Verification items for the finished model (mm, model axes). Round coordinates to 2 decimals unless told otherwise and drop trailing zeros. Order: outer loops, then holes, each group sorted by start corner. A loop starts at its lowest first (then second) coordinate and runs counter-clockwise, first axis right, second up. Notation, with made-up numbers: M 86.25,-12.5 L 113.25,-12.5 A22 ccw 113.25,3.5 Z; hole C 52.5,14 d9. An arc over 180 degrees is marked long. One line per item, written item: value. Start each with the question number.
from build123d import *

# Parameters (mm, degrees)
SKETCH_W             = 129
SKETCH_H             = 90
PAD_DEPTH            = 2
SKETCH001_R          = 2.5
POCKET_DEPTH         = 2.001
SKETCH002_R          = 4.375
POCKET001_DEPTH      = 0.02
SKETCH003_R          = 3.25
PAD001_DEPTH         = 8.2
PAD001_DEPTH_BACK    = -2
POCKET002_DEPTH      = 10
POCKET002_DEPTH_BACK = -5
SKETCH005_W          = 3.16625
SKETCH005_H          = 2
POCKET003_DEPTH      = 45.001
POCKET004_DEPTH      = 53.251


with BuildPart() as part:
    # Sketch → Pad (new body)
    with BuildSketch(Plane.XZ):
        Rectangle(SKETCH_W, SKETCH_H)
    extrude(amount=PAD_DEPTH)

    # Sketch001 → Pocket (cut, through all)
    with BuildSketch(Plane.XZ):
        with Locations((55, 40)):
            Circle(SKETCH001_R)
        with Locations((-55, 40)):
            Circle(SKETCH001_R)
        with Locations((55, -40)):
            Circle(SKETCH001_R)
        with Locations((-55, -40)):
            Circle(SKETCH001_R)
    extrude(amount=POCKET_DEPTH, mode=Mode.SUBTRACT)

    # Sketch002 → Pocket001 (cut)
    with BuildSketch(Plane.XZ):
        with Locations((55, 40)):
            Circle(SKETCH002_R)
        with Locations((-55, 40)):
            Circle(SKETCH002_R)
        with Locations((55, -40)):
            Circle(SKETCH002_R)
        with Locations((-55, -40)):
            Circle(SKETCH002_R)
    extrude(amount=POCKET001_DEPTH, mode=Mode.SUBTRACT)

    # Sketch003 → Pad001 (join, two sides)
    with BuildSketch(Plane.XZ) as pad001_sk:
        with Locations((-15, 40)):
            Circle(SKETCH003_R)
        with BuildLine():
            ThreePointArc((24.25, 50), (21, 53.25), (17.75, 50))
            Line((17.75, 50), (17.75, 40))
            ThreePointArc((17.75, 40), (21, 36.75), (24.25, 40))
            Line((24.25, 40), (24.25, 50))
        make_face()
        with BuildLine():
            ThreePointArc((-13.23, 1.47), (-16.48, 4.72), (-19.73, 1.47))
            Line((-19.73, 1.47), (-19.73, -8.53))
            ThreePointArc((-19.73, -8.53), (-16.48, -11.78), (-13.23, -8.53))
            Line((-13.23, -8.53), (-13.23, 1.47))
        make_face()
        with BuildLine():
            ThreePointArc((-10.58, -30.33), (-13.83, -27.08), (-17.08, -30.33))
            Line((-17.08, -30.33), (-17.08, -40.33))
            ThreePointArc((-17.08, -40.33), (-13.83, -43.58), (-10.58, -40.33))
            Line((-10.58, -40.33), (-10.58, -30.33))
        make_face()
        with BuildLine():
            ThreePointArc((24.25, -12.15), (21, -8.9), (17.75, -12.15))
            Line((17.75, -12.15), (17.75, -22.15))
            ThreePointArc((17.75, -22.15), (21, -25.4), (24.25, -22.15))
            Line((24.25, -22.15), (24.25, -12.15))
        make_face()
    extrude(amount=-PAD001_DEPTH)
    extrude(pad001_sk.sketch, amount=-PAD001_DEPTH_BACK)

    # Sketch004 → Pocket002 (cut, two sides)
    with BuildSketch(Plane.XZ) as pocket002_sk:
        with BuildLine():
            ThreePointArc((22.6, 50), (21, 51.6), (19.4, 50))
            Line((19.4, 50), (19.4, 40))
            ThreePointArc((19.4, 40), (21, 38.4), (22.6, 40))
            Line((22.6, 40), (22.6, 50))
        make_face()
        with BuildLine():
            ThreePointArc((-14.88, 1.47), (-16.48, 3.07), (-18.08, 1.47))
            Line((-18.08, 1.47), (-18.08, -8.53))
            ThreePointArc((-18.08, -8.53), (-16.48, -10.13), (-14.88, -8.53))
            Line((-14.88, -8.53), (-14.88, 1.47))
        make_face()
        with BuildLine():
            ThreePointArc((-12.23, -30.33), (-13.83, -28.73), (-15.43, -30.33))
            Line((-15.43, -30.33), (-15.43, -40.33))
            ThreePointArc((-15.43, -40.33), (-13.83, -41.93), (-12.23, -40.33))
            Line((-12.23, -40.33), (-12.23, -30.33))
        make_face()
        with BuildLine():
            ThreePointArc((22.6, -12.15), (21, -10.55), (19.4, -12.15))
            Line((19.4, -12.15), (19.4, -22.15))
            ThreePointArc((19.4, -22.15), (21, -23.75), (22.6, -22.15))
            Line((22.6, -22.15), (22.6, -12.15))
        make_face()
    extrude(amount=-POCKET002_DEPTH, mode=Mode.SUBTRACT)
    extrude(pocket002_sk.sketch, amount=-POCKET002_DEPTH_BACK, mode=Mode.SUBTRACT)

    # Sketch005 → Pocket003 (cut, through all)
    with BuildSketch(Plane.XY):
        with Locations((20.983125, 7.2)):
            Rectangle(SKETCH005_W, SKETCH005_H)
    extrude(amount=-POCKET003_DEPTH, mode=Mode.SUBTRACT)

    # Sketch005 → Pocket004 (cut, through all)
    with BuildSketch(Plane.XY):
        with Locations((20.983125, 7.2)):
            Rectangle(SKETCH005_W, SKETCH005_H)
    extrude(amount=POCKET004_DEPTH, mode=Mode.SUBTRACT)


solid = part.part
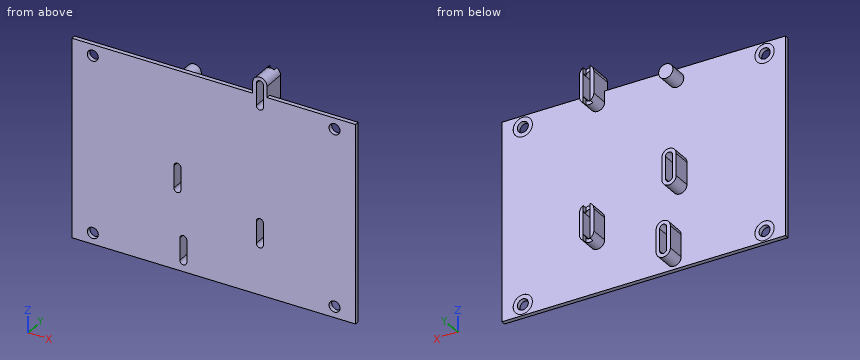
1. Section check C-C (z = 28). Record the cut outline in (x, y), and give its area (3 significant figures).
2. Scan lines: line 1 along X through (y, z) = (-1.35, -40); line 2 along X through (y, z) = (-1, 40); line 3 along X through (y, z) = (1.5, 47). Record each from-to range of solid material in increasing order.
3. Section check D-D (x = 1). Record the cut outline in (y, z).
4. Section check A-A (x = 55). Record the cut outline in (y, z) (3 decimals), and give its area (3 significant figures).
5. Section check B-B (x = 21). Record the cut outline in (y, z).
6. Depth check by flat-ended pin: pin 1 (1.6 mm diameter, centred on x = -32.5, y = -0.5, fed in from +Z); pin 2 (4.5 mm diameter, centred on x = -55.5, z = -38.5, fed in from +Y); pin 3 (0.6 mm diameter, centred on y = 7.5, z = -10, fed in from -X); pin 4 (5 mm diameter, centred on y = 3, z = 11, fed in from -X). Enter the tip coordinate at first touch or a pass-through.
Geometry check:
1. outline: M -64.5,-2 L 64.5,-2 L 64.5,0 L -64.5,0 Z
1. area: 258 mm²
2. line 1: x = -64.5 to -57.5, -52.5 to -15.43, -12.23 to 52.5, 57.5 to 64.5
2. line 2: x = -64.5 to -57.5, -52.5 to 19.4, 22.6 to 52.5, 57.5 to 64.5
2. line 3: x = 17.75 to 19.4, 22.6 to 24.25
3. outline: M -2,-45 L 0,-45 L 0,45 L -2,45 Z
4. outline: M -2,-45 L 0,-45 L 0,-44.375 L -0.02,-44.375 L -0.02,-42.5 L -2,-42.5 Z; M -2,-37.5 L -0.02,-37.5 L -0.02,-35.625 L 0,-35.625 L 0,35.625 L -0.02,35.625 L -0.02,37.5 L -2,37.5 Z; M -2,42.5 L -0.02,42.5 L -0.02,44.375 L 0,44.375 L 0,45 L -2,45 Z
4. area: 160 mm²
5. outline: M -2,-45 L 0,-45 L 0,-25.4 L 6.2,-25.4 L 6.2,-23.75 L -2,-23.75 Z; M -2,-10.55 L 6.2,-10.55 L 6.2,-8.9 L 0,-8.9 L 0,36.75 L 6.2,36.75 L 6.2,38.4 L -2,38.4 Z; M -2,51.6 L 6.2,51.6 L 6.2,53.25 L -2,53.25 Z
6. pin 1: stops at z = 45
6. pin 2: stops at y = -0.02
6. pin 3: stops at x = -19.51
6. pin 4: passes through
